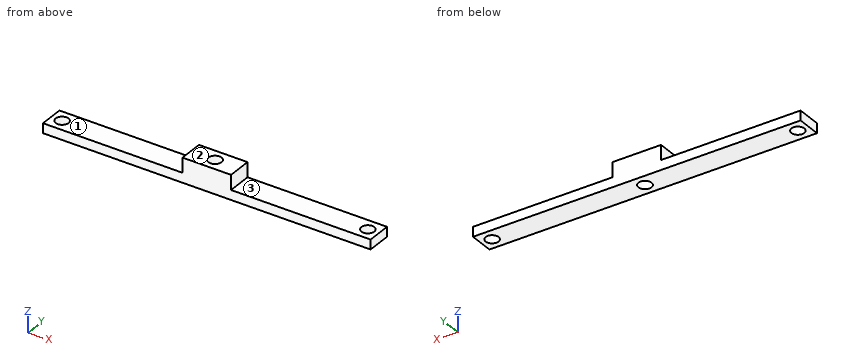
from build123d import *

# Parameters (mm, degrees)
SKETCH1_W             = 85.725
SKETCH1_H             = 6.35
BOSS_EXTRUDE1_DEPTH   = 6.40182
SKETCH2_W             = 36.5125
SKETCH2_H             = 6.35
CUT_EXTRUDE1_DEPTH    = 3.86182
M3_CLEARANCE_HOLE1_D  = 3.4
F_8_32_TAPPED_HOLE1_D = 3.4544


with BuildPart() as part:
    # Sketch1 → Boss-Extrude1 (new body)
    with BuildSketch(Plane.XY):
        Rectangle(SKETCH1_W, SKETCH1_H)
    extrude(amount=BOSS_EXTRUDE1_DEPTH)

    # Sketch2 → Cut-Extrude1 (cut)
    with BuildSketch(Plane.XY.offset(6.40182)):
        with Locations((24.60625, 0)):
            Rectangle(SKETCH2_W, SKETCH2_H)
    cut_extrude1 = extrude(amount=-CUT_EXTRUDE1_DEPTH, mode=Mode.SUBTRACT)

    # M3 Clearance Hole1 (through all)
    with Locations(Plane.XY.offset(2.54)):
        with Locations((40.005, 0)):
            m3_clearance_hole1 = Hole(M3_CLEARANCE_HOLE1_D / 2)

    # Mirror2: Cut-Extrude1, M3 Clearance Hole1 across plane
    add(cut_extrude1.mirror(Plane(origin=(0, 0, 0), x_dir=(0, 0, 1), z_dir=(1, 0, 0))), mode=Mode.SUBTRACT)
    add(m3_clearance_hole1.mirror(Plane(origin=(0, 0, 0), x_dir=(0, 0, 1), z_dir=(1, 0, 0))), mode=Mode.SUBTRACT)

    # #8-32 Tapped Hole1 (through all)
    with Locations(Plane.XY.offset(6.40182)):
        with Locations((0, 0)):
            Hole(F_8_32_TAPPED_HOLE1_D / 2)


solid = part.part
Here's how the part is built. I have some questions about the finished solid (model axes, mm). Face numbers are marked on the shaded views. A direction names the side the tool comes from. Coordinates: 2 decimals unless noted, no trailing zeros. Write each loop counter-clockwise with the first axis right and the second up, starting at its lowest first coordinate (ties: lowest second). Pieces come first, ordered by that corner, then holes.
Item 1: On a 3-axis mill with a long thin cutter (end or side, diameter ignored), from which of +Z, -Z, +X, -X, +Y, -Y can I reach the whole of each face in a straight line? I mean the marked faces 1, 2 and 3. Say none if no direction works.
Item 2: I want a section at C-C on y = 1. Write out the boundary of the cut face in (x, z).
Item 3: I want a section at A-A on x = 0. Write out the boundary of the cut face in (y, z) (3 decimals).
Item 4: If I drill on line 1 (Y direction, x = 0, z = 1.5) (3 decimals); line 2 (X direction, y = -0.75, z = 1); line 3 (Z direction, x = 10, y = 1.75), over which ranges is the centre line in solid material (lowest first)?
Item 5: I want a section at B-B on z = 1.75. Write out the boundary of the cut face in (x, y) (1 decimal).
Item 6: Will these pins go through, and if not, where does the flat tip stop? pin 1 (1.2 mm diameter, centred on y = 1, z = 4, fed in from +X); pin 2 (3 mm diameter, centred on x = 21.5, y = 1.5, fed in from -Z); pin 3 (1.9 mm diameter, centred on x = 23.5, y = -0.5, fed in from +Z); pin 4 (1.2 mm diameter, centred on y = -0.5, z = 4, fed in from -X).
Item 7: I want a section at D-D on x = -20.5. Write out the boundary of the cut face in (y, z) (3 decimals).
Findings below:
1. face 1: +Z, -X, +Y, -Y
1. face 2: +Z, +X, -X, +Y, -Y
1. face 3: +Z, +X, +Y, -Y
2. outline: (-42.86, 0) - (-41.38, 0) - (-41.38, 2.54) - (-42.86, 2.54) - close; (-38.63, 0) - (-1.41, 0) - (-1.41, 6.4) - (-6.35, 6.4) - (-6.35, 2.54) - (-38.63, 2.54) - close; (1.41, 0) - (38.63, 0) - (38.63, 2.54) - (6.35, 2.54) - (6.35, 6.4) - (1.41, 6.4) - close; (41.38, 0) - (42.86, 0) - (42.86, 2.54) - (41.38, 2.54) - close
3. outline: (-3.175, 0) - (-1.727, 0) - (-1.727, 6.402) - (-3.175, 6.402) - close; (1.727, 0) - (3.175, 0) - (3.175, 6.402) - (1.727, 6.402) - close
4. line 1: y = -3.175 to -1.727, 1.727 to 3.175
4. line 2: x = -42.86 to -41.53, -38.48 to -1.56, 1.56 to 38.48, 41.53 to 42.86
4. line 3: z = 0 to 2.54
5. outline: (-42.9, -3.2) - (42.9, -3.2) - (42.9, 3.2) - (-42.9, 3.2) - close; hole circle Ø3.4 at (-40, 0); hole circle Ø3.5 at (0, 0); hole circle Ø3.4 at (40, 0)
6. pin 1: stops at x = 6.35
6. pin 2: stops at z = 0
6. pin 3: stops at z = 2.54
6. pin 4: stops at x = -6.35
7. outline: (-3.175, 0) - (3.175, 0) - (3.175, 2.54) - (-3.175, 2.54) - close
